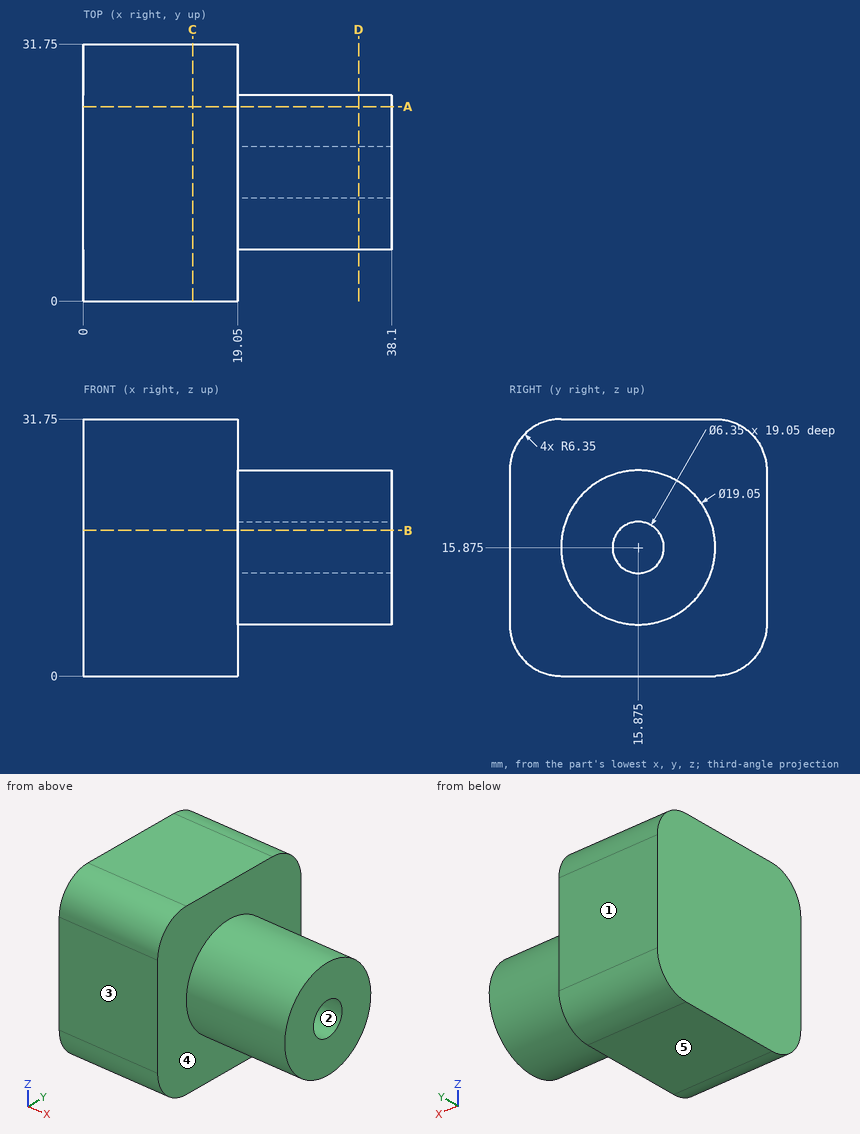
Source: three-view drawing plus pictorial views. Frame: mm from the lowest corner of the part. A direction names the side the tool comes from. Round coordinates to 2 decimals unless told otherwise and drop trailing zeros. Order: outer loops, then holes, each group sorted by start corner. A loop starts at its lowest first (then second) coordinate and runs counter-clockwise, first axis right, second up. Notation, with made-up numbers: (-20, -12.75) - (-12, -12.75) arc R14 ccw to (-12, 6.25) - close; hole circle Ø4 at (-25.5, 41.25). An arc over 180 degrees is marked (long way). Answer in a Markdown table with one row per item.
Item 1: Section query A-A (y = 24). Return the cut outline in (x, z), then the cut area to 3 significant figures.
Model answer:
| item | result |
|---|---|
| outline | (0, 0) - (19.05, 0) - (19.05, 10.9) - (38.1, 10.9) - (38.1, 20.85) - (19.05, 20.85) - (19.05, 31.75) - (0, 31.75) - close |
| area | 794 mm² |
Item 2: Line query: line 1 (X direction, y = 20, z = 5); line 2 (Y direction, x = 27.5, z = 13); line 3 (Y direction, x = 8.5, z = 27). Output: solid intervals per line, ascending.
Model answer:
| item | result |
|---|---|
| line 1 | x = 0 to 19.05 |
| line 2 | y = 6.79 to 14.53, 17.22 to 24.96 |
| line 3 | y = 0.2 to 31.55 |
Item 3: Mould query, pull axis Y, two halves, no side actions, for the marked faces 1, 2 and 3. Classes: released by +Y, released by -Y, zero draft, split by the parting line, or undercut.
Model answer:
| item | result |
|---|---|
| face 1 | released by +Y |
| face 2 | undercut |
| face 3 | released by -Y |
Item 4: Section query D-D (x = 34). Return the cut outline in (y, z) (3 decimals), then the cut area to 3 significant figures.
Model answer:
| item | result |
|---|---|
| outline | circle Ø19.05 at (15.875, 15.875); hole circle Ø6.35 at (15.875, 15.875) |
| area | 253 mm² |
Item 5: Reachability of the marked faces 4 and 5 from +Z, -Z, +X, -X, +Y, -Y: full face, straight path, thin tool, end or side. Return the list, or none.
Model answer:
| item | result |
|---|---|
| face 4 | +X |
| face 5 | -Z, +X, -X, +Y, -Y |
Item 6: Section query C-C (x = 13.5). Return the cut outline in (y, z), then the cut area to 3 significant figures.
Model answer:
| item | result |
|---|---|
| outline | (0, 6.35) arc R6.35 ccw to (6.35, 0) - (25.4, 0) arc R6.35 ccw to (31.75, 6.35) - (31.75, 25.4) arc R6.35 ccw to (25.4, 31.75) - (6.35, 31.75) arc R6.35 ccw to (0, 25.4) - close |
| area | 973 mm² |
Item 7: Pin query (flat end, axial travel): pin 1 (4 mm diameter, centred on y = 15.875, z = 15.875, fed in from +X); pin 2 (1 mm diameter, centred on x = 10, y = 28.5, fed in from +Z). Return the tip coordinate at first contact, or that it passes through.
Model answer:
| item | result |
|---|---|
| pin 1 | stops at x = 19.05 |
| pin 2 | stops at z = 31.19 |
Item 8: Section query B-B (z = 18). Return the cut outline in (x, y), then the cut area to 3 significant figures.
Model answer:
| item | result |
|---|---|
| outline | (0, 0) - (19.05, 0) - (19.05, 6.59) - (38.1, 6.59) - (38.1, 13.52) - (19.05, 13.52) - (19.05, 18.23) - (38.1, 18.23) - (38.1, 25.16) - (19.05, 25.16) - (19.05, 31.75) - (0, 31.75) - close |
| area | 869 mm² |
